Read the model definition and answer for the solid it produces. Units are mm, in the model's axes. Face numbers are marked on the shaded views. Coordinates: 2 decimals unless noted, no trailing zeros. Write each loop counter-clockwise with the first axis right and the second up, starting at its lowest first coordinate (ties: lowest second). Pieces come first, ordered by that corner, then holes. Notation, with made-up numbers: (63.25, 25) -> (101.25, 25) arc R18 cw to (101.25, 48) -> close; hole circle Ø2 at (-6.5, 48.5). An arc over 180 degrees is marked (long way). One line per item, written item: value. Start each with the question number.
1. For a pull along Y with two mould halves and no side action, classify the marked faces 1, 2, 3 and 4 as pulls with the +Y half, pulls with the -Y half, needs draft (parallel to the pull), parting line crosses it, or undercut.
2. Find section A-A, the plane z = 31.5. Write down the section's boundary in (x, y).
3. Find section D-D, the plane y = 21.5. Write down the section's boundary in (x, z).
4. Find section B-B, the plane x = 3.75. State how many separate pieces and enclosed holes the cut face has, and give its area (3 significant figures).
5. Consider line 1 along X through (y, z) = (19.5, 9.5); line 2 along Y through (x, z) = (2.75, 4.5); line 3 along X through (y, z) = (6.5, 20). Determine where each line is inside the solid, lowest interval first.
6. Given P1, Ø6, axis at y = 8.5, z = 7, coming from the +X side; P2, Ø3, axis at x = 2, z = 15.5, coming from the +Y side; P3, Ø3, axis at x = 2, z = 24.5, coming from the -Y side, each flat-ended and moving along its own axis, determine where each tip first touches the part or whether it passes through.
7. Find section C-C, the plane y = 16. Write down the section's boundary in (x, z).
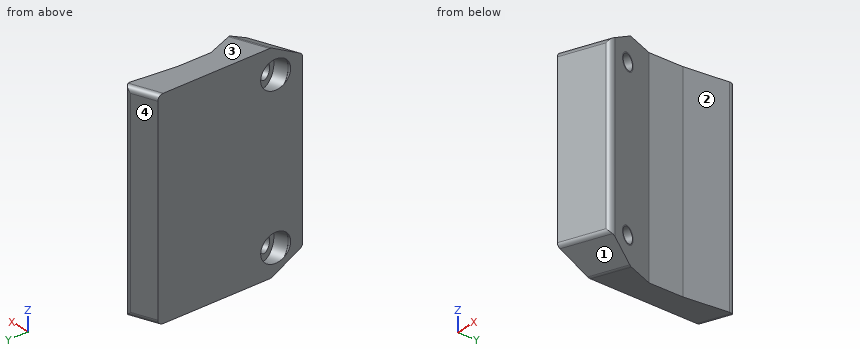
```python
from build123d import *

# Parameters (mm, degrees)
EXTRUDE_L_DEPTH        = 40.640000266
SKETCH_506_R           = 1.642286764
EXTRUDE_A_DEPTH        = 8.205424
SKETCH_6_R             = 1.647216999
EXTRUDE_B_DEPTH        = 8.205424
SKETCH_66_R            = 2.75
CUT_EXTRUDE_2755_DEPTH = 51.448100318
CUT_EXTRUDE_2790_REACH = 51.787
FILLET_3_R             = 1


with BuildPart() as part:
    # 主L型: read off the stored shape, not the designer's step
    # 主L型 outline → 主L型 (new body)
    with BuildSketch(Plane.XY):
        Polygon((0, 28.473390503), (0, 0), (8.845423506, 3.395440187), (4.726521328, 14.125546488), (4.773897119, 20.740741864), (5.951057155, 30.762189648), align=None)
    extrude(amount=EXTRUDE_L_DEPTH)

    # Sketch 506 → 螺丝台A (add)
    with BuildSketch(Plane(origin=(8.845423506, 3.395440187, 0), x_dir=(0, 0, -1), z_dir=(0.9335804184498224, 0.3583679705094393, 0))):
        with Locations((-5.045565417, 4.946234453)):
            Circle(SKETCH_506_R)
    extrude(amount=-EXTRUDE_A_DEPTH)

    # 螺丝穿出面<6> → 螺丝台B (add)
    with BuildSketch(Plane(origin=(8.845423506, 3.395440187, 0), x_dir=(0, 0, -1), z_dir=(0.9335804184498224, 0.3583679705094393, 0))):
        with Locations((-35.594637562, 4.953875303)):
            Circle(SKETCH_6_R)
    extrude(amount=-EXTRUDE_B_DEPTH)

    # 草图64 → 螺丝A M2.5 凹头盖螺钉的柱形沉头孔14 (revolve, cut)
    with BuildSketch(Plane(origin=(-0.587571577, 5.072586706, 5.045565417), x_dir=(0.3583679705094393, -0.9335804184498224, 0), z_dir=(0, 0, 1))):
        Polygon((0, 0), (0, 18.012790366), (1.45, 18.012790366), (1.45, 2.5), (2.75, 2.5), (2.75, 0.025), (2.775, 0), align=None)
    revolve(axis=Axis((-6.515807234, 2.796950093, 5.045565417), (0.9335804184498225, 0.3583679705094394, 0)), mode=Mode.SUBTRACT)

    # 草图65 → 螺丝B M2.5 凹头盖螺钉的柱形沉头孔15 (revolve, cut)
    with BuildSketch(Plane(origin=(-0.590309813, 5.079720054, 35.594637562), x_dir=(0.3583679705094393, -0.9335804184498224, 0), z_dir=(0, 0, 1))):
        Polygon((0, 0), (0, 18.012790366), (1.45, 18.012790366), (1.45, 2.5), (2.75, 2.5), (2.75, 0.025), (2.775, 0), align=None)
    revolve(axis=Axis((-6.51854547, 2.804083441, 35.594637562), (0.9335804184498225, 0.35836797050943936, 0)), mode=Mode.SUBTRACT)

    # 草图66 → Cut-Extrude 2755 (cut, through all)
    with BuildSketch(Plane(origin=(3.518951472, 1.350799002, 0), x_dir=(0, 0, 1), z_dir=(-0.9335804184498225, -0.3583679705094393, 0))):
        with Locations(Location((5.045565417, 4.946234453, 0), (0, 0, 270))):
            Circle(SKETCH_66_R)
        with Locations(Location((35.594637562, 4.953875303, 0), (0, 0, 270))):
            Circle(SKETCH_66_R)
    extrude(amount=CUT_EXTRUDE_2755_DEPTH, mode=Mode.SUBTRACT)

    # Cut-Extrude 2790: up to this plane
    cut_extrude_2790_end = Plane(origin=(0, 28.473390503, 72.648652673), z_dir=(1, 0, 0))
    # 螺丝穿出面<7> → Cut-Extrude 2790 (cut, up to the surface)
    with BuildSketch(Plane(origin=(8.845423506, 3.395440187, 0), x_dir=(0, 0, -1), z_dir=(0.9335804184498224, 0.3583679705094393, 0)), mode=Mode.PRIVATE) as cut_extrude_2790_sk1:
        Polygon((0, 5.796717469), (-3.346571729, 0), (0, 0), align=None)
    cut_extrude_2790_tool1 = split(extrude(cut_extrude_2790_sk1.sketch, amount=-CUT_EXTRUDE_2790_REACH, mode=Mode.PRIVATE), bisect_by=cut_extrude_2790_end, keep=Keep.BOTH, mode=Mode.PRIVATE)
    cut_extrude_2790 = cut_extrude_2790_tool1.solids().sort_by_distance((8.152971, 5.199341, 1.115524))[0]
    add(cut_extrude_2790, mode=Mode.SUBTRACT)

    # 镜向6: Cut-Extrude 2790 across plane
    add(cut_extrude_2790.mirror(Plane(origin=(0, 0, 20.320000133), x_dir=(1, 0, 0), z_dir=(0, 0, -1))), mode=Mode.SUBTRACT)

    # 圆角3
    fillet_3_edges = [part.edges().sort_by_distance(p)[0] for p in [
        (5.951057155, 30.762189648, 20.320000133),
        (2.975528577, 29.617790076, 0),
        (2.975528577, 29.617790076, 40.640000266),
        (4.422711753, 1.697720093, 3.346571729),
        (3.384032816, 7.508133528, 0),
        (8.845423506, 3.395440187, 20.320000133),
        (3.384032816, 7.508133528, 40.640000266),
        (4.422711753, 1.697720093, 37.293428537),
    ]]
    fillet(fillet_3_edges, radius=FILLET_3_R)


solid = part.part
```
Answer block:
1. face 1: pulls with the -Y half
1. face 2: undercut
1. face 3: needs draft
1. face 4: pulls with the +Y half
2. outline: (0, 0) -> (7.91, 3.04) arc R1 ccw to (8.49, 4.33) -> (4.73, 14.13) -> (4.77, 20.74) -> (5.76, 29.12) arc R1 ccw to (4.41, 30.17) -> (0, 28.47) -> close
3. outline: (0, 0) -> (4.86, 0) -> (4.86, 40.64) -> (0, 40.64) -> close
4. separate pieces: 1
4. enclosed holes: 2
4. area: 1,120 mm2
5. line 1: x = 0 to 4.77
5. line 2: y = 1.06 to 4.91, 7.79 to 29.53
5. line 3: x = 0 to 7.65
6. P1: stops at x = 8.04
6. P2: stops at y = 29.82
6. P3: stops at y = 0.19
7. outline: (0, 0) -> (4.74, 0) -> (4.74, 40.64) -> (0, 40.64) -> close
